Part model, mm, in its own coordinate system. A direction names the side the tool comes from. Coordinates: 2 decimals unless noted, no trailing zeros. Write each loop counter-clockwise with the first axis right and the second up, starting at its lowest first coordinate (ties: lowest second). Pieces come first, ordered by that corner, then holes. Notation, with made-up numbers: M -6.5,-14 L 30.5,-14 A37 cw 30.5,24 Z; hole C -9,17.25 d2. An arc over 180 degrees is marked long. Use a Markdown table: item, result. Add a question column.
Q1. Mould opens along Y. For faces 4 (the cylindrical face through (-48.37, -12.67, -2.46)), 5 (the flat face through (6.1, 2.1, -9)), 6 (the cylindrical face through (1.172, 8.923, -6.972)), 7 (the cylindrical face through (43.16, -25.24, -2.46)) say: released by +Y, released by -Y, zero draft, split by the parting line, or undercut.
Q2. Slice it at B-B on x = -20. Count the separate pieces of the cut face and the enclosed holes in it, then the cut area to 3 significant figures.
Q3. Pin check, flat tips, straight feed: pin 1 Ø4.5 at (x, z) = (-1, -7) entering from +Y; pin 2 Ø2 at (x, z) = (-1, -6.5) entering from -Y; pin 3 Ø1.5 at (y, z) = (-12, -2) entering from -X. Stop position of each tip, or through.
Q4. Wall check: L1, parallel to Y at x = 36, z = -3.75; L2, parallel to Y at x = 0, z = -3.85; L3, parallel to X at y = 37, z = -1.5. Give the ranges that are in metal, low to high. Write a range as from..to.
Q5. Tool access for faces 1 (the flat face through (4, 0, 0)), 2 (the flat face through (11.63, -24.54, -2.46)), 3 (the flat face through (-3, 0, -5)): list every direction of +Z, -Z, +X, -X, +Y, -Y with a clear straight run to the whole face (end or side of a thin tool).
Q6. Slice it at A-A on z = -7.25. Write the cut outline in (x, y), then the cut area to 3 significant figures.
from build123d import *

# Parameters (mm, degrees)
SKETCH1_R           = 60
BOSS_EXTRUDE1_DEPTH = 5
CUT_EXTRUDE2_DEPTH  = 5
SKETCH9_R           = 1.5
SKETCH10_R          = 9
BOSS_EXTRUDE2_DEPTH = 4
CUT_EXTRUDE4_DEPTH  = 4
SKETCH12_R          = 2.5
CUT_EXTRUDE5_DEPTH  = 6


with BuildPart() as part:
    # Sketch1 → Boss-Extrude1 (new body)
    with BuildSketch(Plane.XY):
        Circle(SKETCH1_R)
    extrude(amount=-BOSS_EXTRUDE1_DEPTH)

    # Sketch7 → Cut-Extrude2 (cut)
    with BuildSketch(Plane.XY):
        with BuildLine():
            ThreePointArc((-4.786620503, -49.770355275), (12.911635843, -48.304137088), (28.981073455, -40.744292624))
            Line((28.981073455, -40.744292624), (-6.221076455, -7.872795103))
            Line((-6.221076455, -7.872795103), (-4.786620503, -49.770355275))
        make_face()
        with BuildLine():
            Line((49.303279175, -8.317852043), (1.167941456, -9.965872152))
            Line((1.167941456, -9.965872152), (31.8083039, -38.577607534))
            ThreePointArc((31.8083039, -38.577607534), (43.286088156, -25.026277633), (49.303279175, -8.317852043))
        make_face()
        with BuildLine():
            Line((40.744292624, 28.981073455), (7.872795103, -6.221076455))
            Line((7.872795103, -6.221076455), (49.770355275, -4.786620503))
            ThreePointArc((49.770355275, -4.786620503), (49.94255582, -2.396063049), (50, 0))
            ThreePointArc((50, 0), (47.629899387, 15.211597037), (40.744292624, 28.981073455))
        make_face()
        with BuildLine():
            Line((9.965872152, 1.167941456), (38.577607534, 31.8083039))
            ThreePointArc((38.577607534, 31.8083039), (25.026277633, 43.286088156), (8.317852043, 49.303279175))
            Line((8.317852043, 49.303279175), (9.965872152, 1.167941456))
        make_face()
        with BuildLine():
            Line((6.221076455, 7.872795103), (4.786620503, 49.770355275))
            ThreePointArc((4.786620503, 49.770355275), (-12.911635843, 48.304137088), (-28.981073455, 40.744292624))
            Line((-28.981073455, 40.744292624), (6.221076455, 7.872795103))
        make_face()
        with BuildLine():
            Line((-1.167941456, 9.965872152), (-31.8083039, 38.577607534))
            ThreePointArc((-31.8083039, 38.577607534), (-43.286088156, 25.026277633), (-49.303279175, 8.317852043))
            Line((-49.303279175, 8.317852043), (-1.167941456, 9.965872152))
        make_face()
        with BuildLine():
            ThreePointArc((-49.770355275, 4.786620503), (-48.304137088, -12.911635843), (-40.744292624, -28.981073455))
            Line((-40.744292624, -28.981073455), (-7.872795103, 6.221076455))
            Line((-7.872795103, 6.221076455), (-49.770355275, 4.786620503))
        make_face()
        with BuildLine():
            ThreePointArc((-38.577607534, -31.8083039), (-25.026277633, -43.286088156), (-8.317852043, -49.303279175))
            Line((-8.317852043, -49.303279175), (-9.965872152, -1.167941456))
            Line((-9.965872152, -1.167941456), (-38.577607534, -31.8083039))
        make_face()
    extrude(amount=-CUT_EXTRUDE2_DEPTH, mode=Mode.SUBTRACT)

    # Sketch9 → Cut-Revolve3 (revolve, cut)
    with BuildSketch(Plane(origin=(0, 0, 0), x_dir=(1, 0, 0), z_dir=(0, 1, 0))):
        with Locations((-60, 2.5)):
            Circle(SKETCH9_R)
    revolve(axis=Axis((0, 0, -92.148103423), (0, 0, 1)), mode=Mode.SUBTRACT)

    # Sketch10 → Boss-Extrude2 (add)
    with BuildSketch(Plane(origin=(0, 0, -5), x_dir=(-1, 0, 0), z_dir=(0, 0, -1))):
        Circle(SKETCH10_R)
    extrude(amount=BOSS_EXTRUDE2_DEPTH)

    # Sketch11 → Cut-Extrude4 (cut)
    with BuildSketch(Plane(origin=(0, 0, -9), x_dir=(-1, 0, 0), z_dir=(0, 0, -1))):
        Polygon((7, 0), (3.5, 6.062177826), (-3.5, 6.062177826), (-7, 0), (-3.5, -6.062177826), (3.5, -6.062177826), align=None)
    extrude(amount=-CUT_EXTRUDE4_DEPTH, mode=Mode.SUBTRACT)

    # Sketch12 → Cut-Extrude5 (cut, through all)
    with BuildSketch(Plane(origin=(0, 0, -5), x_dir=(-1, 0, 0), z_dir=(0, 0, -1))):
        Circle(SKETCH12_R)
    extrude(amount=-CUT_EXTRUDE5_DEPTH, mode=Mode.SUBTRACT)


solid = part.part
Recorded:
| question | item | result |
|---|---|---|
| 1 | face 4 | undercut |
| 1 | face 5 | zero draft |
| 1 | face 6 | split by the parting line |
| 1 | face 7 | undercut |
| 2 | separate pieces | 5 |
| 2 | enclosed holes | 0 |
| 2 | area | 167 mm² |
| 3 | pin 1 | y = 60 |
| 3 | pin 2 | y = -9 |
| 3 | pin 3 | x = -57.95 |
| 4 | L1 | -46.96..-34.7, -8.77..-5.26, 23.9..29.05, 34.7..46.96 |
| 4 | L2 | -59.35..-50, -13.68..-2.5, 2.5..13.68, 50..59.35 |
| 4 | L3 | -45.8..-33.63, -30.12..-24.97, 5.22..8.74, 33.63..45.8 |
| 5 | face 1 | +Z, +X, -X, +Y, -Y |
| 5 | face 2 | +Z, -Z |
| 5 | face 3 | -Z |
| 6 | outline | C 0,0 d18; hole M -7,0 L -3.5,-6.06 L 3.5,-6.06 L 7,0 L 3.5,6.06 L -3.5,6.06 Z |
| 6 | area | 127 mm² |
